from build123d import *

# Parameters (mm, degrees)
ESQUISSE1_W             = 40.9
ESQUISSE1_H             = 5
ESQUISSE1_W_2           = 8
ESQUISSE1_H_2           = 30
ESQUISSE1_R             = 2
BOSS_EXTRU_1_DEPTH      = 11
ESQUISSE2_R             = 1.8
ENL_V_MAT_EXTRU_1_DEPTH = 9
ESQUISSE3_W             = 56.9
ESQUISSE3_H             = 30
ENL_V_MAT_EXTRU_2_DEPTH = 1.5


with BuildPart() as part:
    # Esquisse1 → Boss.-Extru.1 (new body)
    # profile 1 of 3: a face of its own
    with BuildSketch(Plane.XY):
        with Locations((28.45, 2.5)):
            Rectangle(ESQUISSE1_W, ESQUISSE1_H)
    # profile 2 of 3: a face of its own
    with BuildSketch(Plane.XY):
        with Locations((4, 15)):
            Rectangle(ESQUISSE1_W_2, ESQUISSE1_H_2)
        with Locations((4.15, 15)):
            Circle(ESQUISSE1_R, mode=Mode.SUBTRACT)
        with Locations((4.15, 25)):
            Circle(ESQUISSE1_R, mode=Mode.SUBTRACT)
    # profile 3 of 3: a face of its own
    with BuildSketch(Plane.XY):
        Polygon((48.9, 5), (48.9, 0), (56.9, 0), (56.9, 30), (48.9, 30), align=None)
        with Locations((52.75, 15)):
            Circle(ESQUISSE1_R, mode=Mode.SUBTRACT)
        with Locations((52.75, 25)):
            Circle(ESQUISSE1_R, mode=Mode.SUBTRACT)
    extrude(amount=BOSS_EXTRU_1_DEPTH)

    # Esquisse2 → Enlèv. mat.-Extru.1 (cut)
    with BuildSketch(Plane.XZ):
        with Locations((18.45, 4)):
            Circle(ESQUISSE2_R)
        with Locations((38.45, 4)):
            Circle(ESQUISSE2_R)
    extrude(amount=-ENL_V_MAT_EXTRU_1_DEPTH, mode=Mode.SUBTRACT)

    # Esquisse3 → Enlèv. mat.-Extru.2 (cut)
    with BuildSketch(Plane.XY.offset(11)):
        with Locations((28.45, 15)):
            Rectangle(ESQUISSE3_W, ESQUISSE3_H)
    extrude(amount=-ENL_V_MAT_EXTRU_2_DEPTH, mode=Mode.SUBTRACT)


solid = part.part
Model file for the job. Use its own axes, mm. A direction names the side the tool comes from. Give positions to 0.01 mm unless a question says otherwise; leave off trailing zeros. Loops run counter-clockwise (first coordinate to the right, second up) from the corner with the lowest first, then second, coordinate; pieces in that order, holes last. Notation, with made-up numbers: (62.25, 28) -> (119.25, 28) arc R16 ccw to (119.25, 53) -> close; hole circle Ø7 at (-3, 47.5). An arc over 180 degrees is marked (long way). Use a Markdown table: item, result. Add a question column.
(1) Drop flat-ended pins along their axis: pin 1 Ø3 at (x, z) = (38.45, 4) entering from +Y; pin 2 Ø4 at (x, z) = (21.5, 5) entering from +Y. Give the stop position or say it passes through.
(2) Slice it at B-B on y = 19.25. List the corners of the cut face in (x, z).
(3) Slice it at C-C on z = 4. List the corners of the cut face in (x, y).
(4) Slice it at A-A on x = 52.75. List the corners of the cut face in (y, z).
(5) Tool access for faces 5 (the flat face through (28, 0, 5)), 6 (the flat face through (8, 17, 5)): list every direction of +Z, -Z, +X, -X, +Y, -Y with a clear straight run to the whole face (end or side of a thin tool).
(6) Mould opens along Z. For faces 1 (the flat face through (28, 4, 9.5)), 2 (the flat face through (48.9, 18, 5)), 3 (the flat face through (28, 4, 0)), 4 (the cylindrical face through (16.65, 2.46, 4.08)) say: +Z half, -Z half, draft (parallel to the pull), parting line (faces both ways), or undercut.
(7) Wall check: line 1 along Y through (x, z) = (52.75, 2); line 2 along X through (y, z) = (15, 5.25); line 3 along X through (y, z) = (22.5, 5.75). Give the ranges that are in metal, low to high.
(8) Slice it at D-D on y = 25. List the corners of the cut face in (x, z).
Filled sheet:
| question | item | result |
|---|---|---|
| 1 | pin 1 | through |
| 1 | pin 2 | y = 5 |
| 2 | outline | (0, 0) -> (8, 0) -> (8, 9.5) -> (0, 9.5) -> close; (48.9, 0) -> (56.9, 0) -> (56.9, 9.5) -> (48.9, 9.5) -> close |
| 3 | outline | (0, 0) -> (16.65, 0) -> (16.65, 5) -> (8, 5) -> (8, 30) -> (0, 30) -> close; (20.25, 0) -> (36.65, 0) -> (36.65, 5) -> (20.25, 5) -> close; (40.25, 0) -> (56.9, 0) -> (56.9, 30) -> (48.9, 30) -> (48.9, 5) -> (40.25, 5) -> close; hole circle Ø4 at (4.15, 15); hole circle Ø4 at (4.15, 25); hole circle Ø4 at (52.75, 15); hole circle Ø4 at (52.75, 25) |
| 4 | outline | (0, 0) -> (13, 0) -> (13, 9.5) -> (0, 9.5) -> close; (17, 0) -> (23, 0) -> (23, 9.5) -> (17, 9.5) -> close; (27, 0) -> (30, 0) -> (30, 9.5) -> (27, 9.5) -> close |
| 5 | face 5 | +Z, -Z, +X, -X, -Y |
| 5 | face 6 | +Z, -Z, +Y |
| 6 | face 1 | +Z half |
| 6 | face 2 | draft |
| 6 | face 3 | -Z half |
| 6 | face 4 | undercut |
| 7 | line 1 | 0 to 13, 17 to 23, 27 to 30 |
| 7 | line 2 | 0 to 2.15, 6.15 to 8, 48.9 to 50.75, 54.75 to 56.9 |
| 7 | line 3 | 0 to 8, 48.9 to 56.9 |
| 8 | outline | (0, 0) -> (2.15, 0) -> (2.15, 9.5) -> (0, 9.5) -> close; (6.15, 0) -> (8, 0) -> (8, 9.5) -> (6.15, 9.5) -> close; (48.9, 0) -> (50.75, 0) -> (50.75, 9.5) -> (48.9, 9.5) -> close; (54.75, 0) -> (56.9, 0) -> (56.9, 9.5) -> (54.75, 9.5) -> close |
